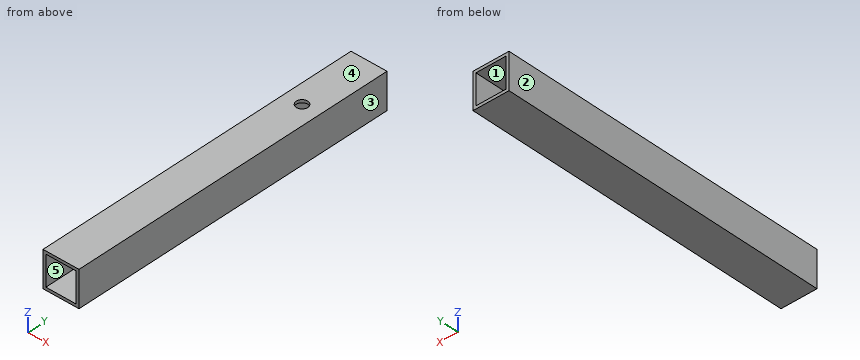
```python
from build123d import *

# Parameters (mm, degrees)
F0_W     = 25
F0_H     = 25
F0_W_2   = 21
F0_H_2   = 21
F1_DEPTH = 230
F3_D     = 8
F3_DEPTH = 5


with BuildPart() as f1:
    # F0 (on Front) → F1 (new body)
    with BuildSketch(Plane.XZ):
        with Locations((12.5, 12.5)):
            Rectangle(F0_W, F0_H)
        with Locations((12.5, 12.5)):
            Rectangle(F0_W_2, F0_H_2, mode=Mode.SUBTRACT)
    extrude(amount=F1_DEPTH)

    # F3
    with Locations(Plane.XY.offset(25)):
        with Locations((12.5, -50)):
            Hole(F3_D / 2, depth=F3_DEPTH)


solid = f1.part
```
Work out the finished part from the listing and answer in its coordinate system (mm). Face numbers are marked on the shaded views. A direction names the side the tool comes from. Coordinates: 2 decimals unless noted, no trailing zeros. Write each loop counter-clockwise with the first axis right and the second up, starting at its lowest first coordinate (ties: lowest second). Pieces come first, ordered by that corner, then holes.
Q1. Which of the six approach directions +Z, -Z, +X, -X, +Y, -Y give full straight-line access (tool end or side, diameter ignored) to the marked faces 1 and 2?
Q2. A cutting plane is placed at C-C, the plane y = -137. Give the vertices of the cut face in (x, z).
Q3. A cutting plane is placed at D-D, the plane y = -50. Give the vertices of the cut face in (x, z).
Q4. A cutting plane is placed at B-B, the plane z = 4. Give the vertices of the cut face in (x, y).
Q5. Determine the mould class of the marked faces 3, 4 and 5 for opening direction X: released by +X, released by -X, zero draft, split by the parting line, or undercut.
Q6. Find the intervals of material crossed by line 1 (Z direction, x = 21.5, y = -70.5); line 2 (Y direction, x = 12.5, z = 24.2), in increasing order.
Q7. A cutting plane is placed at A-A, the plane x = 12.5. Give the vertices of the cut face in (y, z), then the cut area to 3 significant figures.
Findings below:
1. face 1: +Y, -Y
1. face 2: +Z, -Z, -X, +Y, -Y
2. outline: (0, 0) - (25, 0) - (25, 25) - (0, 25) - close; hole (2, 2) - (23, 2) - (23, 23) - (2, 23) - close
3. outline: (0, 0) - (25, 0) - (25, 25) - (16.5, 25) - (16.5, 23) - (23, 23) - (23, 2) - (2, 2) - (2, 23) - (8.5, 23) - (8.5, 25) - (0, 25) - close
4. outline: (0, -230) - (2, -230) - (2, 0) - (0, 0) - close; (23, -230) - (25, -230) - (25, 0) - (23, 0) - close
5. face 3: released by +X
5. face 4: zero draft
5. face 5: undercut
6. line 1: z = 0 to 2, 23 to 25
6. line 2: y = -230 to -54, -46 to 0
7. outline: (-230, 0) - (0, 0) - (0, 2) - (-230, 2) - close; (-230, 23) - (-54, 23) - (-54, 25) - (-230, 25) - close; (-46, 23) - (0, 23) - (0, 25) - (-46, 25) - close
7. area: 904 mm2
